Design review of the part shown in the three views and the two pictorial views. Dimensions are in mm from the part's minimum x, y and z. Coordinates: 2 decimals unless noted, no trailing zeros. Use a Markdown table: item, result. Add a question column.
Q1. Take a section at A-A on x = 158.75. Count the separate pieces of the cut face and the enclosed holes in it, plus the area to 3 significant figures.
Q2. For probe 1 along Y at (x, z) = (29.5, 5.25) (1 decimal); probe 2 along X at (y, z) = (87, 3) (1 decimal); probe 3 along X at (y, z) = (28, 2) (1 decimal), list the stretches that pass through material, from the lowest coordinate up.
Q3. Clearance check with flat-ended pins moving along their axes: pin 1 Ø19.5 at (x, y) = (28.575, 22.225) entering from -Z; pin 2 Ø13.5 at (x, y) = (158.75, 152.4) entering from +Z. State where each tip first meets the part, or that it passes through.
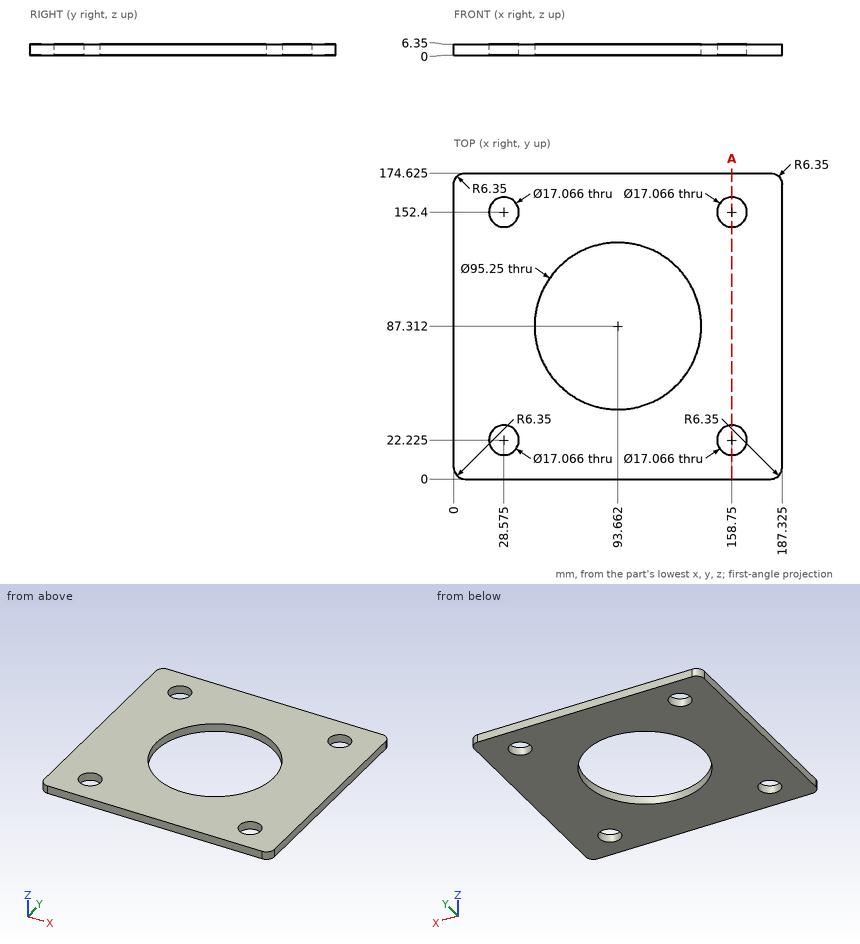
Answer list:
| question | item | result |
|---|---|---|
| 1 | separate pieces | 3 |
| 1 | enclosed holes | 0 |
| 1 | area | 892 mm² |
| 2 | probe 1 | 0 to 13.7, 30.7 to 143.9, 160.9 to 174.6 |
| 2 | probe 2 | 0 to 46, 141.3 to 187.3 |
| 2 | probe 3 | 0 to 22.3, 34.9 to 152.5, 165 to 187.3 |
| 3 | pin 1 | z = 0 |
| 3 | pin 2 | through |
